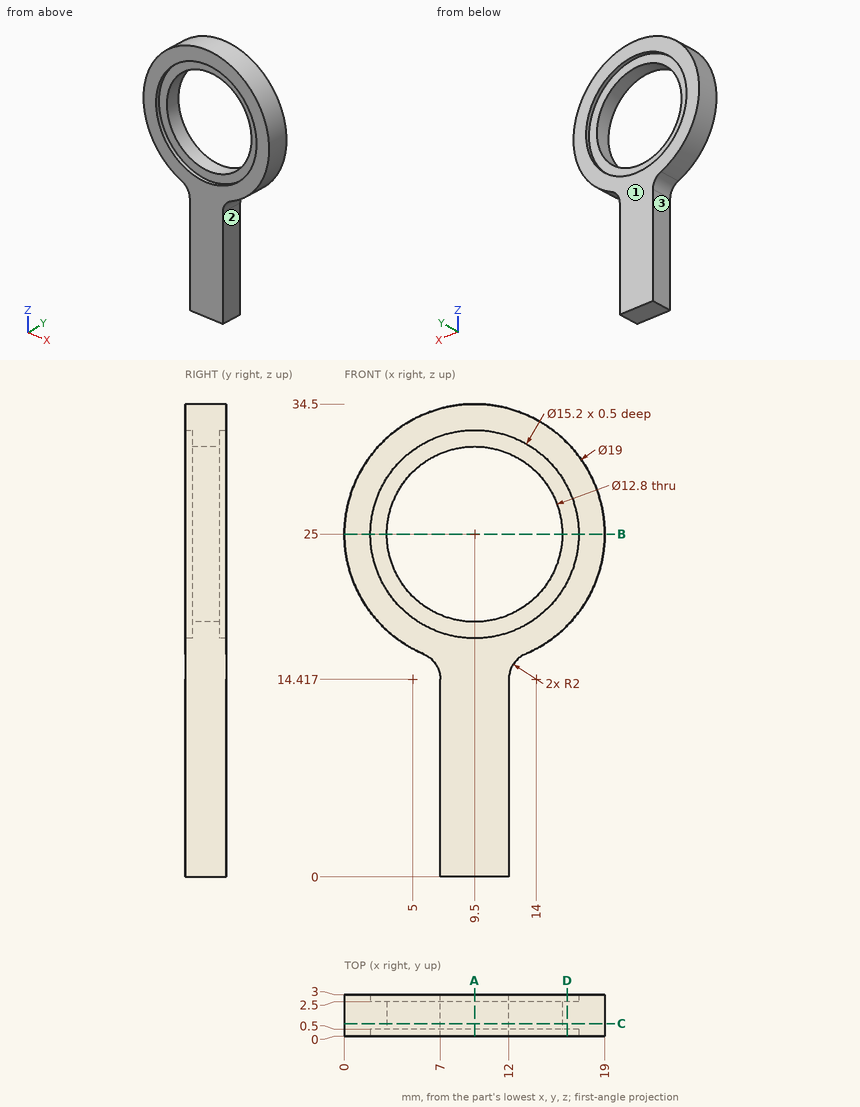
Can you work these out from the drawing? Everything is in mm from the part's minimum corner. A direction names the side the tool comes from. Give positions to 0.01 mm unless a question says otherwise; leave off trailing zeros. Order: outer loops, then holes, each group sorted by start corner. A loop starts at its lowest first (then second) coordinate and runs counter-clockwise, first axis right, second up.
Item 1: If we section it at C-C, the plane y = 0.9: Write out the boundary of the cut face in (x, z), plus the area to 3 significant figures.
Item 2: If we section it at D-D, the plane x = 16.25: Write out the boundary of the cut face in (y, z), plus the area to 3 significant figures.
Item 3: If we section it at A-A, the plane x = 9.5: Write out the boundary of the cut face in (y, z), plus the area to 3 significant figures.
Item 4: If we section it at B-B, the plane z = 25: Write out the boundary of the cut face in (x, y).
Item 5: For the marked faces 1, 2 and 3, which set-ups out of +Z, -Z, +X, -X, +Y, -Y let a thin tool reach every point of the face, with its end or its side?
Item 6: I'm going to push flat-ended pins straight in: pin 1 (1.5 mm diameter, centred on y = 1, z = 7.5, fed in from +X); pin 2 (1.5 mm diameter, centred on y = 2, z = 11, fed in from -X); pin 3 (1.5 mm diameter, centred on y = 1, z = 27, fed in from +X). Where does each tip first touch, or does it pass through?
Item 7: I need wall thicknesses on line 1 (X direction, y = 0.1, z = 25); line 2 (X direction, y = 1, z = 4.5); line 3 (Z direction, x = 9, y = 2.55). Which ranges of each line are inside material? Lowest first, please.
Values:
1. outline: (5.78, 16.26) arc R2 cw to (7, 14.42) - (7, 0) - (12, 0) - (12, 14.42) arc R2 cw to (13.22, 16.26) arc R9.5 ccw (long way) to start; hole circle Ø12.8 at (9.5, 25)
1. area: 234 mm2
2. outline: (0, 18.32) - (3, 18.32) - (3, 21.51) - (2.5, 21.51) - (2.5, 28.49) - (3, 28.49) - (3, 31.68) - (0, 31.68) - (0, 28.49) - (0.5, 28.49) - (0.5, 21.51) - (0, 21.51) - close
2. area: 33.1 mm2
3. outline: (0, 0) - (3, 0) - (3, 17.4) - (2.5, 17.4) - (2.5, 18.6) - (0.5, 18.6) - (0.5, 17.4) - (0, 17.4) - close; (0, 32.6) - (0.5, 32.6) - (0.5, 31.4) - (2.5, 31.4) - (2.5, 32.6) - (3, 32.6) - (3, 34.5) - (0, 34.5) - close
3. area: 62.7 mm2
4. outline: (0, 0) - (1.9, 0) - (1.9, 0.5) - (3.1, 0.5) - (3.1, 2.5) - (1.9, 2.5) - (1.9, 3) - (0, 3) - close; (15.9, 0.5) - (17.1, 0.5) - (17.1, 0) - (19, 0) - (19, 3) - (17.1, 3) - (17.1, 2.5) - (15.9, 2.5) - close
5. face 1: +Z, -Z, +X, -X, +Y
5. face 2: -Z, +X, +Y, -Y
5. face 3: -Z, -X, +Y, -Y
6. pin 1: stops at x = 12
6. pin 2: stops at x = 7
6. pin 3: stops at x = 18.92
7. line 1: x = 0 to 1.9, 17.1 to 19
7. line 2: x = 7 to 12
7. line 3: z = 0 to 17.42, 32.58 to 34.49
